```python
from build123d import *


with BuildPart() as part:
    # Sketch1 → Revolve1 (revolve)
    with BuildSketch(Plane.XY, mode=Mode.PRIVATE) as revolve1_sk:
        with BuildLine():
            Line((-15.5, 0), (-17.5, 0))
            Line((-17.5, 0), (-17.5, 100))
            ThreePointArc((-17.5, 100), (-16.53803894, 102.011461655), (-14.675685538, 103.237425306))
            ThreePointArc((-14.675685538, 103.237425306), (-16.718615549, 106.063714958), (-13.402842077, 104.983380513))
            Line((-13.402842077, 104.983380513), (-13.402842077, 97.692354136))
            Line((-13.402842077, 97.692354136), (-4.333255578, 97.692354136))
            Line((-4.333255578, 97.692354136), (-4.333255578, 103.999749208))
            Line((-4.333255578, 103.999749208), (-1.5875, 103.999749208))
            Line((-1.5875, 103.999749208), (-1.5875, 108.999749208))
            Line((-1.5875, 108.999749208), (0, 108.999749208))
            Line((0, 108.999749208), (0, 2.753698387))
            ThreePointArc((0, 2.753698387), (-7.871353994, 2.059925785), (-15.5, 0))
        make_face()
    revolve(revolve1_sk.sketch.rotate(Axis((0, -1000, 0), (0, 1, 0)), 270), axis=Axis((0, -1000, 0), (0, 1, 0)))


solid = part.part
```
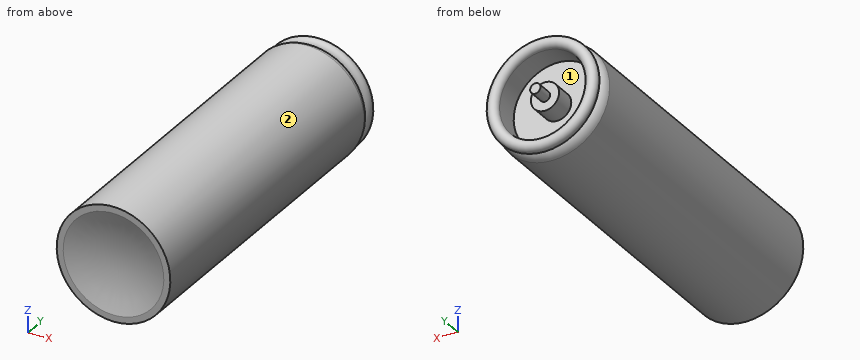
Model file for the job. Use its own axes, mm. Face numbers are marked on the shaded views. Give positions to 0.01 mm unless a question says otherwise; leave off trailing zeros. Loops run counter-clockwise (first coordinate to the right, second up) from the corner with the lowest first, then second, coordinate; pieces in that order, holes last. Notation, with made-up numbers: (8, 2) -> (42, 2) arc R26 cw to (42, 18) -> close; hole circle Ø8 at (31.5, 76.25). An arc over 180 degrees is marked (long way). Use CSV: the item, a comma, the result in double quotes. Start each with the question number.
1) Slice it at A-A on z = 0. Give the cut face in (x, y), plus the area to 3 significant figures.
2) Mould opens along X. For the marked faces 1 and 2 say: released by +X, released by -X, zero draft, split by the parting line, or undercut.
3) Wall check: line 1 (X direction, y = 99.75, z = 0); line 2 (X direction, y = 101.5, z = 0); line 3 (Y direction, x = -2, z = 10). Give the ranges that are in metal, low to high.
4) Slice it at B-B on x = 0. Give the cut face in (y, z), plus the area to 3 significant figures.
5) Flat gauge pins, fed straight in: pin 1 Ø1 at (x, z) = (3, 6.5) entering from +Y; pin 2 Ø2 at (y, z) = (41, 9) entering from -X; pin 3 Ø1 at (x, z) = (-1.5, 12) entering from -Y. Where does each tip first touch, or does it go through?
6) Slice it at C-C on y = 11. Give the cut face in (x, z), plus the area to 3 significant figures.
Computed values:
1,outline,"(-17.5, 0) -> (-15.5, 0) arc R45 cw to (15.5, 0) -> (17.5, 0) -> (17.5, 100) arc R4.16 ccw to (14.68, 103.24) arc R1.83 ccw (long way) to (13.4, 104.98) -> (13.4, 97.69) -> (4.33, 97.69) -> (4.33, 104) -> (1.59, 104) -> (1.59, 109) -> (-1.59, 109) -> (-1.59, 104) -> (-4.33, 104) -> (-4.33, 97.69) -> (-13.4, 97.69) -> (-13.4, 104.98) arc R1.83 ccw (long way) to (-14.68, 103.24) arc R4.16 ccw to (-17.5, 100) -> close"
1,area,"3,490 mm^2"
2,face 1,"undercut"
2,face 2,"split by the parting line"
3,line 1,"x = -17.5 to -13.4, -4.33 to 4.33, 13.4 to 17.5"
3,line 2,"x = -16.92 to -13.4, -4.33 to 4.33, 13.4 to 16.92"
3,line 3,"y = 1.58 to 97.69"
4,outline,"(0, -17.5) -> (100, -17.5) arc R4.16 ccw to (103.24, -14.68) arc R1.83 ccw (long way) to (104.98, -13.4) -> (97.69, -13.4) -> (97.69, -4.33) -> (104, -4.33) -> (104, -1.59) -> (109, -1.59) -> (109, 1.59) -> (104, 1.59) -> (104, 4.33) -> (97.69, 4.33) -> (97.69, 13.4) -> (104.98, 13.4) arc R1.83 ccw (long way) to (103.24, 14.68) arc R4.16 ccw to (100, 17.5) -> (0, 17.5) -> (0, 15.5) arc R45 cw to (0, -15.5) -> close"
4,area,"3,490 mm^2"
5,pin 1,"stops at y = 97.69"
5,pin 2,"stops at x = -15.56"
5,pin 3,"stops at y = 0.96"
6,outline,"circle Ø35 at (0, 0)"
6,area,"962 mm^2"
